from build123d import *

# Parameters (mm, degrees)
SKETCH1_W           = 25
SKETCH1_H           = 5
BOSS_EXTRUDE1_DEPTH = 10
SKETCH2_W           = 25
SKETCH2_H           = 5
BOSS_EXTRUDE2_DEPTH = 40
SKETCH3_W           = 7
SKETCH3_H           = 2.5
BOSS_EXTRUDE3_DEPTH = 2.5


with BuildPart() as part:
    # Sketch1 → Boss-Extrude1 (new body)
    with BuildSketch(Plane(origin=(0, 0, 0), x_dir=(1, 0, 0), z_dir=(0, 1, 0))):
        Rectangle(SKETCH1_W, SKETCH1_H)
    extrude(amount=BOSS_EXTRUDE1_DEPTH)

    # Sketch2 → Boss-Extrude2 (add)
    with BuildSketch(Plane.XY.offset(2.5)):
        with Locations((0, 7.5)):
            Rectangle(SKETCH2_W, SKETCH2_H)
    extrude(amount=BOSS_EXTRUDE2_DEPTH)

    # Sketch3 → Boss-Extrude3 (add)
    with BuildSketch(Plane.XZ.offset(-5)):
        with Locations((-0.17068016, 37.447744065)):
            Rectangle(SKETCH3_W, SKETCH3_H)
    extrude(amount=BOSS_EXTRUDE3_DEPTH)


solid = part.part
Model file for the job. Use its own axes, mm. A direction names the side the tool comes from. Round coordinates to 2 decimals unless told otherwise and drop trailing zeros. Loops run counter-clockwise (first coordinate to the right, second up) from the corner with the lowest first, then second, coordinate; pieces in that order, holes last. Notation, with made-up numbers: (6.5, -4.75) -> (11.5, -4.75) arc R21 cw to (11.5, 19.25) -> close; hole circle Ø6 at (-4.5, 14). An arc over 180 degrees is marked (long way). Answer as CSV lines item,"result". Start each with the question number.
1) Slice it at D-D (x = -5). List the corners of the cut face in (y, z).
2) Tool access for faces 1 (the face through (0, 2, 2.5)), 2 (the face through (-3.671, 4, 37)), 3 (the face through (0, 2.5, 37)): list every direction of +Z, -Z, +X, -X, +Y, -Y with a clear straight run to the whole face (end or side of a thin tool).
3) Slice it at A-A (y = 4.25). List the corners of the cut face in (x, z).
4) Slice it at B-B (x = 1.5). List the corners of the cut face in (y, z), plus the area to 3 significant figures.
5) Pin check, flat tips, straight feed: P1, Ø2, axis at x = 1.5, z = 37, coming from the -Y side; P2, Ø10, axis at x = 7.5, z = 32, coming from the -Y side; P3, Ø0.8, axis at y = 3.5, z = 38, coming from the -X side. Stop position of each tip, or through.
6) Probe line 1 along Y through (x, z) = (2.25, 11); line 2 along Z through (x, y) = (10.75, 4.25). List the from-to ranges inside material, lowest first.
7) Slice it at C-C (z = 29). List the corners of the cut face in (x, y), plus the area to 3 significant figures.
8) Mould opens along Z. For faces 4 (the face through (3.329, 4, 37)), 5 (the face through (0, 5, -2.5)), 6 (the face through (0, 5, 22)) say: +Z half, -Z half, draft (parallel to the pull), parting line (faces both ways), or undercut.
Filled in:
1,outline,"(0, -2.5) -> (10, -2.5) -> (10, 42.5) -> (5, 42.5) -> (5, 2.5) -> (0, 2.5) -> close"
2,face 1,"+X, -X, -Y"
2,face 2,"+Z, -X, -Y"
2,face 3,"+Z, +X, -X, -Y"
3,outline,"(-12.5, -2.5) -> (12.5, -2.5) -> (12.5, 2.5) -> (-12.5, 2.5) -> close; (-3.67, 36.2) -> (3.33, 36.2) -> (3.33, 38.7) -> (-3.67, 38.7) -> close"
4,outline,"(0, -2.5) -> (10, -2.5) -> (10, 42.5) -> (5, 42.5) -> (5, 38.7) -> (2.5, 38.7) -> (2.5, 36.2) -> (5, 36.2) -> (5, 2.5) -> (0, 2.5) -> close"
4,area,"256 mm2"
5,P1,"stops at y = 2.5"
5,P2,"stops at y = 5"
5,P3,"stops at x = -3.67"
6,line 1,"y = 5 to 10"
6,line 2,"z = -2.5 to 2.5"
7,outline,"(-12.5, 5) -> (12.5, 5) -> (12.5, 10) -> (-12.5, 10) -> close"
7,area,"125 mm2"
8,face 4,"draft"
8,face 5,"-Z half"
8,face 6,"undercut"
